```python
from build123d import *

# Parameters (mm, degrees)
F0_R     = 2.75
F1_DEPTH = 5
F3_DEPTH = 12


with BuildPart() as f1:
    # F0 (on Top) → F1 (new body)
    with BuildSketch(Plane.XY):
        with BuildLine():
            ThreePointArc((-16.248869, 5.803167), (-14.221966, 3.210648), (-13.5, 0))
            ThreePointArc((-13.5, 0), (-17.001528, -6.345252), (-24.236593, -6.765683))
            ThreePointArc((-24.236593, -6.765683), (-18.307775, -10.501181), (-13.396906, -15.5))
            Line((-13.396906, -15.5), (13.396906, -15.5))
            ThreePointArc((13.396906, -15.5), (18.307775, -10.501181), (24.236593, -6.765683))
            ThreePointArc((24.236593, -6.765683), (14.670114, -4.022753), (16.248869, 5.803167))
            ThreePointArc((16.248869, 5.803167), (0, 0), (-16.248869, 5.803167))
        make_face()
        with BuildLine():
            ThreePointArc((-24.236593, -6.765683), (-17.001528, -6.345252), (-13.5, 0))
            ThreePointArc((-13.5, 0), (-14.221966, 3.210648), (-16.248869, 5.803167))
            ThreePointArc((-16.248869, 5.803167), (-27.329886, 4.022753), (-24.236593, -6.765683))
        make_face()
        with Locations((-21, 0)):
            Circle(F0_R, mode=Mode.SUBTRACT)
        with BuildLine():
            ThreePointArc((28.5, 0), (24.210648, 6.778034), (16.248869, 5.803167))
            ThreePointArc((16.248869, 5.803167), (14.670114, -4.022753), (24.236593, -6.765683))
            ThreePointArc((24.236593, -6.765683), (27.345252, -3.998472), (28.5, 0))
        make_face()
        with Locations((21, 0)):
            Circle(F0_R, mode=Mode.SUBTRACT)
    extrude(amount=F1_DEPTH)

    # F2 (on face) → F3 (join)
    with BuildSketch(Plane.XY.offset(5)):
        Polygon((13.396906, -6.5), (0, -6.5), (-13.396906, -6.5), (-13.396906, -15.5), (13.396906, -15.5), align=None)
    extrude(amount=F3_DEPTH)


solid = f1.part
```
Design review of the part built by this model. Coordinates are the model's own, in mm. A direction names the side the tool comes from. Give positions to 0.01 mm unless a question says otherwise; leave off trailing zeros. Order: outer loops, then holes, each group sorted by start corner. A loop starts at its lowest first (then second) coordinate and runs counter-clockwise, first axis right, second up. Notation, with made-up numbers: (-13, 12.5) -> (4, 12.5) arc R28 cw to (4, 30.5) -> close; hole circle Ø1 at (29, -21). An arc over 180 degrees is marked (long way). Write each question's results on one line, items separated by ' | '. Start each with the question number.
Q1. Add section C-C on z = 7.25. Give the boundary of the cut face in (x, y).
Q2. Wall thickness on L1, parallel to Z at x = -12.5, y = -1.5; L2, parallel to Y at x = 21, z = 1.05; L3, parallel to X at y = -6.75, z = 10: over which ranges is each line inside the solid? List them lowest first. Write a range as from..to.
Q3. Add section D-D on x = 5.5. Give the boundary of the cut face in (y, z), and give its area (3 significant figures).
Q4. Add section A-A on y = 2. Give the boundary of the cut face in (x, z).
Q5. Mouldability with a two-part tool opening along X and no side actions: class faces 1 (the flat face through (13.397, -11, 11)), 2 (the flat face through (-13.397, -11, 11)), 3 (the cylindrical face through (18.253, 0.121, 2.465)) as +X half, -X half, draft (parallel to the pull), parting line (faces both ways), or undercut.
Q6. Add section B-B on x = 21. Give the boundary of the cut face in (y, z).
Q7. For pin 1 (4 mm diameter, centred on x = 16, y = -4, fed in from +Z); pin 2 (4 mm diameter, centred on y = 0.5, z = 8.5, fed in from -X); pin 3 (6 mm diameter, centred on x = 3, z = 13, fed in from +Y); pin 4 (1 mm diameter, centred on y = 2, z = 5, fed in from +X), all flat-tipped, find the tip position at first contact; note any pin that passes through.
Q8. Machinability: for faces 4 (the flat face through (0, -6.5, 11)), 5 (the flat face through (0, -4, 0)), which of the approach directions +Z, -Z, +X, -X, +Y, -Y give a long, thin tool a straight path to every point of the face, cutting with its end or side? Answer none if there is none.
Found:
1) outline: (-13.4, -15.5) -> (13.4, -15.5) -> (13.4, -6.5) -> (-13.4, -6.5) -> close
2) L1: z = 0..5 | L2: y = -8.57..-2.75, 2.75..7.5 | L3: x = -13.4..13.4
3) outline: (-15.5, 0) -> (0.6, 0) -> (0.6, 5) -> (-6.5, 5) -> (-6.5, 17) -> (-15.5, 17) -> close | area: 188 mm2
4) outline: (-28.23, 0) -> (-22.89, 0) -> (-22.89, 5) -> (-28.23, 5) -> close; (-19.11, 0) -> (-9.93, 0) -> (-9.93, 5) -> (-19.11, 5) -> close; (9.93, 0) -> (19.11, 0) -> (19.11, 5) -> (9.93, 5) -> close; (22.89, 0) -> (28.23, 0) -> (28.23, 5) -> (22.89, 5) -> close
5) face 1: +X half | face 2: -X half | face 3: undercut
6) outline: (-8.57, 0) -> (-2.75, 0) -> (-2.75, 5) -> (-8.57, 5) -> close; (2.75, 0) -> (7.5, 0) -> (7.5, 5) -> (2.75, 5) -> close
7) pin 1: stops at z = 5 | pin 2: passes through | pin 3: stops at y = -6.5 | pin 4: stops at x = 28.35
8) face 4: +Z, +X, -X, +Y | face 5: -Z, +X, -X, +Y, -Y
